Verification items for the finished model (mm, model axes). Face numbers are marked on the shaded views. A direction names the side the tool comes from. Coordinates: 2 decimals unless noted, no trailing zeros. Write item = value, one per line. Start each with the question number.
(1) Mould release check, pull along Z, two halves, no side actions. Record for the marked faces 4, 5 and 6: released by +Z, released by -Z, zero draft, split by the parting line, or undercut.
(2) Set-up check for the marked faces 1, 2 and 3: record each of +Z, -Z, +X, -X, +Y, -Y from which the full face is reachable in a straight line by a thin tool's end or side.
(3) Section check C-C (y = 3.5). State how many separate pieces and enclosed holes the cut face has, plus the area to 3 significant figures.
(4) Gauge pin test, flat ends, axial feed: pin 1 Ø1.5 at (x, y) = (0, 1.5) entering from +Z; pin 2 Ø2.5 at (x, z) = (-4.5, -7.5) entering from +Y; pin 3 Ø2 at (x, y) = (0, 0.5) entering from -Z. Record the tip position at first contact, or that the pin passes through.
(5) Material ranges on probe 1 along X at (y, z) = (-7.75, 11); probe 2 along X at (y, z) = (3.25, 7.5); probe 3 along Z at (x, y) = (-8.5, 1.5), recorded low to high. Write a range as [from, to].
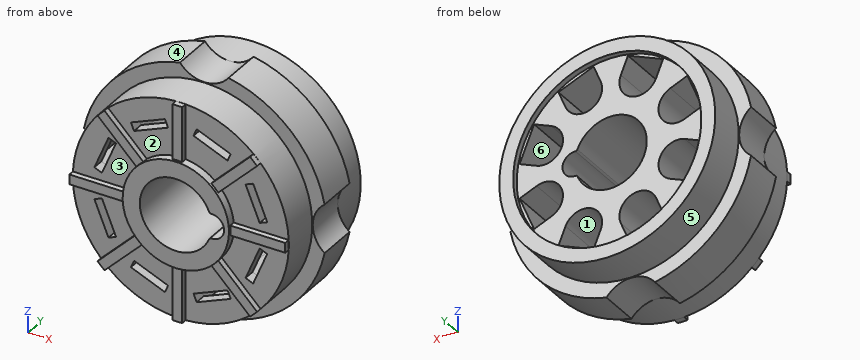
```python
from build123d import *

# Parameters (mm, degrees)
SKETCH2_R           = 11.5
EXTRUDE1_DEPTH      = 0.7
SKETCH4_R           = 6.5
EXTRUDE3_DEPTH      = 1
SKETCH5_W           = 6.714108136
SKETCH5_H           = 1.2
EXTRUDE4_DEPTH      = 0.7
EXTRUDE2_DEPTH      = 24.758998295
EXTRUDE2_DEPTH_BACK = 24.758998295
CIRPATTERN1_COUNT   = 8
EXTRUDE5_DEPTH      = 12.3
EXTRUDE6_DEPTH      = 26.639032743
CIRPATTERN2_COUNT   = 8
SKETCH10_R          = 3.75
EXTRUDE7_DEPTH      = 12.3
CIRPATTERN3_COUNT   = 4


with BuildPart() as part:
    # Sketch1 → Revolve1 (revolve)
    with BuildSketch(Plane.XY, mode=Mode.PRIVATE) as revolve1_sk:
        Polygon((-13.2, 0), (-13.2, 4.7), (0, 4.7), (0, -9.7), (-13.2, -9.7), (-13.2, -5), (-15, -5), (-15, 0), align=None)
    revolve(revolve1_sk.sketch.rotate(Axis((0, 20.644864938, 0), (0, -1, 0)), 270), axis=Axis((0, 20.644864938, 0), (0, -1, 0)))

    # Sketch2 → Extrude1 (cut)
    with BuildSketch(Plane(origin=(0, 4.7, 0), x_dir=(1, 0, 0), z_dir=(0, 1, 0))):
        with Locations(Location((0, 0, 0), (0, 0, 270))):
            Circle(SKETCH2_R)
    extrude(amount=-EXTRUDE1_DEPTH, mode=Mode.SUBTRACT)

    # Sketch4 → Extrude3 (add)
    with BuildSketch(Plane.XZ.offset(9.7)):
        with Locations(Location((0, 0, 0), (0, 0, 270))):
            Circle(SKETCH4_R)
    extrude(amount=EXTRUDE3_DEPTH)

    # Sketch5 → Extrude4 (add)
    with BuildSketch(Plane.XZ.offset(9.7)):
        with Locations((9.829302518, 0)):
            Rectangle(SKETCH5_W, SKETCH5_H)
    extrude4 = extrude(amount=EXTRUDE4_DEPTH)

    # Sketch3 → Extrude2 (cut, two sides: drawn at the far end of the back side and taken through both)
    with BuildSketch(Plane(origin=(0, 0, 0), x_dir=(1, 0, 0), z_dir=(0, 1, 0)).offset(-EXTRUDE2_DEPTH_BACK)):
        with BuildLine():
            ThreePointArc((4.077419355, 1.653678144), (-4.4, 0), (4.077419355, -1.653678144))
            ThreePointArc((4.077419355, -1.653678144), (4.17486489, -1.536726305), (4.322077922, -1.497974683))
            ThreePointArc((4.322077922, -1.497974683), (5.9, 0), (4.322077922, 1.497974683))
            ThreePointArc((4.322077922, 1.497974683), (4.17486489, 1.536726305), (4.077419355, 1.653678144))
        make_face()
    extrude(amount=EXTRUDE2_DEPTH + EXTRUDE2_DEPTH_BACK, mode=Mode.SUBTRACT)

    # CirPattern1: Extrude4 ×8 about axis
    cirpattern1_axis = Axis((0, 0, 0), (0, 1, 0))
    for i in range(1, CIRPATTERN1_COUNT):
        add(extrude4.rotate(cirpattern1_axis, i * 360 / CIRPATTERN1_COUNT))

    # Sketch7 → Extrude5 (cut)
    with BuildSketch(Plane(origin=(0, 4, 0), x_dir=(1, 0, 0), z_dir=(0, 1, 0))):
        with BuildLine():
            Line((9.365323831, 6.395806012), (11.144801791, 2.099766186))
            Line((11.144801791, 2.099766186), (9.04959703, 1.231903958))
            ThreePointArc((9.04959703, 1.231903958), (6.011838137, 2.490184891), (7.27011907, 5.527943784))
            Line((7.27011907, 5.527943784), (9.365323831, 6.395806012))
        make_face()
    extrude5 = extrude(amount=-EXTRUDE5_DEPTH, mode=Mode.SUBTRACT)

    # Sketch9 → Extrude6 (cut, through all)
    with BuildSketch(Plane.XZ.offset(9.7)):
        Polygon((10.561772814, -1.939447092), (8.839697369, -6.096904988), (7.915817836, -5.714221556), (9.637893282, -1.556763659), align=None)
    extrude6 = extrude(amount=-EXTRUDE6_DEPTH, mode=Mode.SUBTRACT)

    # CirPattern2: Extrude5, Extrude6 ×8 about axis
    cirpattern2_axis = Axis((0, 0, 0), (0, 1, 0))
    add([extrude5.rotate(cirpattern2_axis, i * 360 / CIRPATTERN2_COUNT) for i in range(1, CIRPATTERN2_COUNT)], mode=Mode.SUBTRACT)
    add([extrude6.rotate(cirpattern2_axis, i * 360 / CIRPATTERN2_COUNT) for i in range(1, CIRPATTERN2_COUNT)], mode=Mode.SUBTRACT)

    # Sketch10 → Extrude7 (cut)
    with BuildSketch(Plane(origin=(0, 0, 0), x_dir=(1, 0, 0), z_dir=(0, 1, 0))):
        with Locations((17, 0)):
            Circle(SKETCH10_R)
    extrude7 = extrude(amount=-EXTRUDE7_DEPTH, mode=Mode.SUBTRACT)

    # CirPattern3: Extrude7 ×4 about axis
    cirpattern3_axis = Axis((0, 0, 0), (0, 1, 0))
    for i in range(1, CIRPATTERN3_COUNT):
        add(extrude7.rotate(cirpattern3_axis, i * 360 / CIRPATTERN3_COUNT), mode=Mode.SUBTRACT)


solid = part.part
```
Response:
q1.face_4 = released by +Z
q1.face_5 = split by the parting line
q1.face_6 = undercut
q2.face_1 = +Y
q2.face_2 = +Z, -Y
q2.face_3 = -X, -Y
q3.separate_pieces = 1
q3.enclosed_holes = 9
q3.area = 330 mm2
q4.pin_1 = 13.2
q4.pin_2 = 4
q4.pin_3 = -13.35
q5.probe_1 = [-7.3, -2.45], [-2.04, 2.04], [2.45, 7.3]
q5.probe_2 = [-10.86, -5.62], [-1.15, 1.15], [5.62, 10.86]
q5.probe_3 = [-10.1, -6.04], [-1.08, 1.08], [6.04, 10.1]
